Read the model definition and answer for the solid it produces. Units are mm, in the model's axes. Give positions to 0.01 mm unless a question says otherwise; leave off trailing zeros. Order: outer loops, then holes, each group sorted by start corner. A loop starts at its lowest first (then second) coordinate and runs counter-clockwise, first axis right, second up. Notation, with made-up numbers: (8, 77.25) -> (16, 77.25) arc R20 cw to (16, 86.25) -> close; hole circle Ø9 at (57.25, 24.5). An arc over 180 degrees is marked (long way). Use one line per item in the form item = value.
```python
from build123d import *

# Parameters (mm, degrees)
SKETCH1_W           = 303
SKETCH1_H           = 243
SKETCH1_R           = 2
BOSS_EXTRUDE1_DEPTH = 2


with BuildPart() as part:
    # Sketch1 → Boss-Extrude1 (new body)
    with BuildSketch(Plane.XY):
        Rectangle(SKETCH1_W, SKETCH1_H)
        with Locations((85.5, -113.48019802)):
            Circle(SKETCH1_R, mode=Mode.SUBTRACT)
        with Locations((85.5, 113.48019802)):
            Circle(SKETCH1_R, mode=Mode.SUBTRACT)
        with Locations((-85.5, 113.48019802)):
            Circle(SKETCH1_R, mode=Mode.SUBTRACT)
        with Locations((-85.5, -113.48019802)):
            Circle(SKETCH1_R, mode=Mode.SUBTRACT)
        Polygon((94.5, -93.92192355), (86.5, -101.5), (86.5, -96.5), (86.5, 93.5), (94.5, 101.07807645), (94.5, 93.5), align=None, mode=Mode.SUBTRACT)
    extrude(amount=BOSS_EXTRUDE1_DEPTH)


solid = part.part
```
Item 1: The part is cut by section A-A on y = -15. Give the vertices of the cut face in (x, z), and give its area (3 significant figures).
Checks:
outline = (-151.5, 0) -> (86.5, 0) -> (86.5, 2) -> (-151.5, 2) -> close; (94.5, 0) -> (151.5, 0) -> (151.5, 2) -> (94.5, 2) -> close
area = 590 mm²
Item 2: Straight lines are drawn through the part: L1, parallel to Y at x = -85.5, z = 1.4; L2, parallel to X at y = 22.5, z = 1.1; L3, parallel to X at y = -100.5, z = 1.1. For each, find the intervals that lie inside material, in ascending order. Write a range as from..to.
Checks:
L1 = -121.5..-115.48, -111.48..111.48, 115.48..121.5
L2 = -151.5..86.5, 94.5..151.5
L3 = -151.5..86.5, 87.56..151.5
Item 3: The part is cut by section B-B on z = 0.45. Give the vertices of the cut face in (x, y).
Checks:
outline = (-151.5, -121.5) -> (151.5, -121.5) -> (151.5, 121.5) -> (-151.5, 121.5) -> close; hole circle Ø4 at (-85.5, -113.48); hole circle Ø4 at (-85.5, 113.48); hole circle Ø4 at (85.5, -113.48); hole circle Ø4 at (85.5, 113.48); hole (86.5, -101.5) -> (94.5, -93.92) -> (94.5, 101.08) -> (86.5, 93.5) -> close
Item 4: Determine the mould class of faces 1 (the flat face through (90.444, 97.236, 0.986)), 2 (the flat face through (90.556, -97.658, 0.986)), 3 (the flat face through (-2, 2, 0)) for opening direction X: +X half, -X half, draft (parallel to the pull), parting line (faces both ways), or undercut.
Checks:
face_1 = undercut
face_2 = undercut
face_3 = draft
